Answer from the drawing. Dimensions are ordinates in mm from the lowest x, y and z of the part. A direction names the side the tool comes from. Coordinates: 2 decimals unless noted, no trailing zeros. Loops run counter-clockwise (first coordinate to the right, second up) from the corner with the lowest first, then second, coordinate; pieces in that order, holes last. Notation, with made-up numbers: (6, -33) - (10, -33) arc R30 ccw to (10, -3) - close; hole circle Ø5 at (-16.75, 43). An arc over 180 degrees is marked (long way). Use one line per item in the form item = value. Start each with the question number.
1) A cutting plane is placed at D-D (y = 240.5). Give the vertices of the cut face in (x, z).
2) Which of the six approach directions +Z, -Z, +X, -X, +Y, -Y give full straight-line access (tool end or side, diameter ignored) to the marked faces 4, 5 and 6?
3) Consider line 1 (Y direction, x = 147, z = 93); line 2 (Y direction, x = 168, z = 340.5); line 3 (Z direction, x = 62.5, y = 268.5). Determine where each line is inside the solid, lowest interval first.
4) A cutting plane is placed at B-B (x = 70). Give the vertices of the cut face in (y, z).
5) The mould has two halves that part along Y. Classify the marked faces 1, 2 and 3: released by +Y, released by -Y, zero draft, split by the parting line, or undercut.
6) A cutting plane is placed at C-C (z = 265). Give the vertices of the cut face in (x, y), and give its area (3 significant figures).
7) Each of these flat-tipped pins is pushed along its axis until it touches: P1, Ø8, axis at x = 177, y = 114.5, coming from the +Z side; P2, Ø11, axis at x = 4, z = 299, coming from the +Y side; P3, Ø8, axis at y = 295.5, z = 196.5, coming from the +X side. Where does it stop, or does it pass through?
8) A cutting plane is placed at A-A (z = 57.5). Give the vertices of the cut face in (x, y).
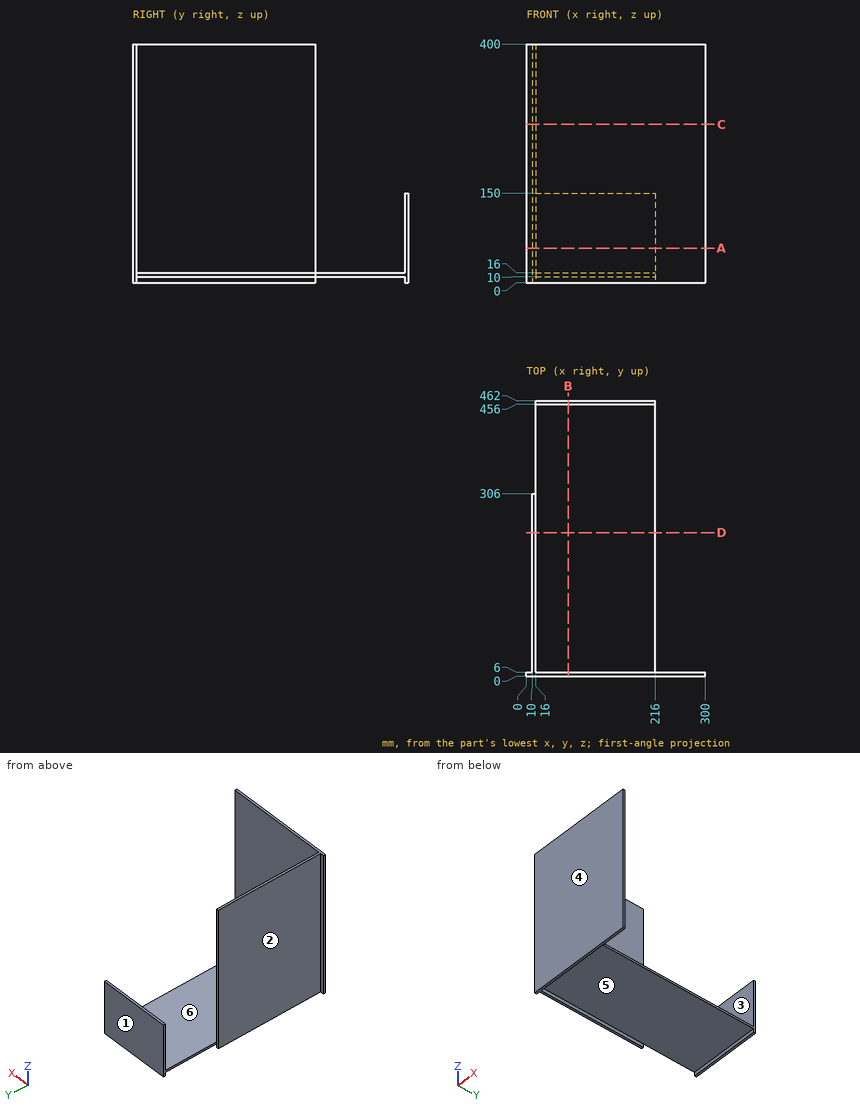
Found:
q1.outline = (10, 0) - (16, 0) - (16, 10) - (216, 10) - (216, 16) - (16, 16) - (16, 400) - (10, 400) - close
q2.face_4 = +Z, -Z, +X, -X, -Y
q2.face_5 = -Z, +X
q2.face_6 = +Z, +X
q3.line_1 = 0 to 6, 456 to 462
q3.line_2 = 0 to 6
q3.line_3 = 10 to 16
q4.outline = (0, 0) - (6, 0) - (6, 10) - (456, 10) - (456, 0) - (462, 0) - (462, 150) - (456, 150) - (456, 16) - (6, 16) - (6, 400) - (0, 400) - close
q5.face_1 = released by +Y
q5.face_2 = zero draft
q5.face_3 = undercut
q6.outline = (0, 0) - (300, 0) - (300, 6) - (16, 6) - (16, 306) - (10, 306) - (10, 6) - (0, 6) - close
q6.area = 3,600 mm^2
q7.P1 = 16
q7.P2 = 6
q7.P3 = 16
q8.outline = (0, 0) - (300, 0) - (300, 6) - (16, 6) - (16, 306) - (10, 306) - (10, 6) - (0, 6) - close; (16, 456) - (216, 456) - (216, 462) - (16, 462) - close
